Here's how the part is built. I have some questions about the finished solid (model axes, mm). Face numbers are marked on the shaded views. A direction names the side the tool comes from. Give positions to 0.01 mm unless a question says otherwise; leave off trailing zeros. Order: outer loops, then holes, each group sorted by start corner. A loop starts at its lowest first (then second) coordinate and runs counter-clockwise, first axis right, second up. Notation, with made-up numbers: M -24.75,24.5 L 18.25,24.5 A10 cw 18.25,31.5 Z; hole C 78.25,6.5 d5. An arc over 180 degrees is marked long. Use one line per item in the form item = value.
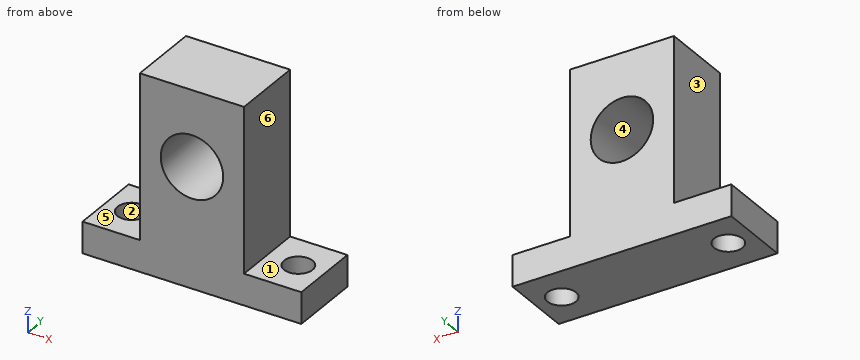
from build123d import *

# Parameters (mm, degrees)
F1_DEPTH = 7
F2_R     = 6
F3_DEPTH = 14.001
F4_R     = 2.75
F5_DEPTH = 6.001


with BuildPart() as f1:
    # F0 (on Front) → F1 (new body, symmetric)
    with BuildSketch(Plane.XZ):
        Polygon((-21, 0), (0, 0), (21, 0), (21, 6), (10, 6), (10, 37.5), (0, 37.5), (-10, 37.5), (-10, 6), (-21, 6), align=None)
    extrude(amount=F1_DEPTH, both=True)

    # F2 (on face) → F3 (cut, through all)
    with BuildSketch(Plane.XZ.offset(7)):
        with Locations((0, 23)):
            Circle(F2_R)
    extrude(amount=-F3_DEPTH, mode=Mode.SUBTRACT)

    # F4 (on face) → F5 (cut, through all)
    with BuildSketch(Plane.XY.offset(6)):
        with Locations((-16, 0)):
            Circle(F4_R)
        with Locations((16, 0)):
            Circle(F4_R)
    extrude(amount=-F5_DEPTH, mode=Mode.SUBTRACT)


solid = f1.part
Q1. I want a section at C-C on z = 23. Write out the boundary of the cut face in (x, y), then the cut area to 3 significant figures.
Found:
outline = M -10,-7 L -6,-7 L -6,7 L -10,7 Z; M 6,-7 L 10,-7 L 10,7 L 6,7 Z
area = 112 mm²
Q2. I want a section at B-B on x = 0. Write out the boundary of the cut face in (y, z), then the cut area to 3 significant figures.
Found:
outline = M -7,0 L 7,0 L 7,17 L -7,17 Z; M -7,29 L 7,29 L 7,37.5 L -7,37.5 Z
area = 357 mm²
Q3. I want a section at A-A on y = 0. Write out the boundary of the cut face in (x, z).
Found:
outline = M -21,0 L -18.75,0 L -18.75,6 L -21,6 Z; M -13.25,0 L 13.25,0 L 13.25,6 L 10,6 L 10,37.5 L -10,37.5 L -10,6 L -13.25,6 Z; M 18.75,0 L 21,0 L 21,6 L 18.75,6 Z; hole C 0,23 d12
Q4. Thinking about a two-plate mould opening in X: for the marked faces 4, 5 and 6, which applies, +X half, -X half, draft (parallel to the pull), parting line (faces both ways), or undercut?
Found:
face_4 = undercut
face_5 = draft
face_6 = +X half
Q5. I'm going to push flat-ended pins straight in: pin 1 Ø3 at (x, y) = (14.5, -1.5) entering from +Z; pin 2 Ø1 at (x, y) = (-4.5, 4.5) entering from -Z; pin 3 Ø7 at (y, z) = (-2.5, 29.5) entering from -X; pin 4 Ø5 at (x, y) = (16, 0) entering from +Z. Where does each tip first touch, or does it pass through?
Found:
pin_1 = 6
pin_2 = 0
pin_3 = -10
pin_4 = through
Q6. I want a section at D-D on y = -5.5. Write out the boundary of the cut face in (x, z).
Found:
outline = M -21,0 L 21,0 L 21,6 L 10,6 L 10,37.5 L -10,37.5 L -10,6 L -21,6 Z; hole C 0,23 d12
Q7. On a 3-axis mill with a long thin cutter (end or side, diameter ignored), from which of +Z, -Z, +X, -X, +Y, -Y can I reach the whole of each face in a straight line? I mean the marked faces 1, 2 and 3. Say none if no direction works.
Found:
face_1 = +Z, +X, +Y, -Y
face_2 = +Z, -Z
face_3 = +Z, -X, +Y, -Y
Q8. I need wall thicknesses on L1, parallel to Y at x = 16, z = 1.9; L2, parallel to Z at x = 19.5, y = -2; L3, parallel to Z at x = -2, y = 0.25. Which ranges of each line are inside material? Lowest first, please.
Found:
L1 = -7 to -2.75, 2.75 to 7
L2 = 0 to 6
L3 = 0 to 17.34, 28.66 to 37.5
